from build123d import *

# Parameters (mm, degrees)
F0_W     = 45
F0_H     = 20
F1_DEPTH = 50
F3_SIZE  = 2
F4_SIZE  = 5
F2_R     = 5
F5_DEPTH = 45
F6_W     = 70
F6_H     = 70
F7_DEPTH = 50
F8_W     = 60
F8_H     = 60
F9_DEPTH = 40


with BuildPart() as f1:
    # F0 (on Top) → F1 (new body)
    with BuildSketch(Plane.XY):
        Rectangle(F0_W, F0_H)
    extrude(amount=F1_DEPTH)

    # F3
    f3_edges = [f1.edges().sort_by_distance(p)[0] for p in [
        (-22.5, -10, 25),
        (-22.5, 10, 25),
        (22.5, -10, 25),
        (22.5, 10, 25),
    ]]
    chamfer(f3_edges, length=F3_SIZE)

    # F4
    f4_edges = [f1.edges().sort_by_distance(p)[0] for p in [
        (0, 10, 0),
        (0, -10, 0),
    ]]
    chamfer(f4_edges, length=F4_SIZE)

    # F2 (on face) → F5 (cut, through all)
    with BuildSketch(Plane(origin=(-22.5, 0, 0), x_dir=(0, -1, 0), z_dir=(-1, 0, 0))):
        with Locations((0, 7)):
            Circle(F2_R)
    extrude(amount=-F5_DEPTH, mode=Mode.SUBTRACT)

    # F6 (on face) → F7 (join)
    with BuildSketch(Plane.XY.offset(50)):
        Rectangle(F6_W, F6_H)
    extrude(amount=F7_DEPTH)

    # F8 (on face) → F9 (cut)
    with BuildSketch(Plane.XY.offset(100)):
        Rectangle(F8_W, F8_H)
    extrude(amount=-F9_DEPTH, mode=Mode.SUBTRACT)


solid = f1.part
Could you check a few things on this model? Use its own coordinates, in mm. A direction names the side the tool comes from. Give positions to 0.01 mm unless a question says otherwise; leave off trailing zeros. Order: outer loops, then holes, each group sorted by start corner. A loop starts at its lowest first (then second) coordinate and runs counter-clockwise, first axis right, second up.
Item 1: If we section it at D-D, the plane y = -19: Write out the boundary of the cut face in (x, z).
Item 2: If we section it at B-B, the plane y = 0: Write out the boundary of the cut face in (x, z).
Item 3: If we section it at C-C, the plane x = -0.5: Write out the boundary of the cut face in (y, z), plus the area to 3 significant figures.
Item 4: I need wall thicknesses on line 1 (Z direction, x = -11, y = 0); line 2 (Y direction, x = -28, z = 79). Which ranges of each line are inside material? Lowest first, please.
Item 5: I'm going to push flat-ended pins straight in: pin 1 (1.5 mm diameter, centred on x = 20, y = 12, fed in from -Z); pin 2 (12 mm diameter, centred on x = 11, z = 30, fed in from +Y); pin 3 (10 mm diameter, centred on x = -21.5, y = -16, fed in from +Z); pin 4 (10 mm diameter, centred on x = 24.5, y = -1.5, fed in from -Z). Where does each tip first touch, or does it pass through?
Item 6: For faces 5 (the face through (22.5, 0, 25)), 6 (the face through (0, 30, 80)), 7 (the face through (0, -10, 27)), 8 (the face through (0, 10, 27)), which set-ups out of +Z, -Z, +X, -X, +Y, -Y let a thin tool reach every point of the face, with its end or its side?
Item 7: If we section it at A-A, the plane z = 7: Write out the boundary of the cut face in (x, y), plus the area to 3 significant figures.
Item 8: If we mould it in two halves opening along Y, with no side actions, what happens to faces 1 (the face through (0, 8, 3)), 2 (the face through (35, 0, 75)), 3 (the face through (0, -30, 80)), 4 (the face through (0, -8, 3))? For each: pulls with the +Y half, pulls with the -Y half, needs draft (parallel to the pull), parting line crosses it, or undercut.
Values:
1. outline: (-35, 50) - (35, 50) - (35, 100) - (30, 100) - (30, 60) - (-30, 60) - (-30, 100) - (-35, 100) - close
2. outline: (-35, 50) - (-22.5, 50) - (-22.5, 12) - (22.5, 12) - (22.5, 50) - (35, 50) - (35, 100) - (30, 100) - (30, 60) - (-30, 60) - (-30, 100) - (-35, 100) - close; (-22.5, 0) - (22.5, 0) - (22.5, 2) - (-22.5, 2) - close
3. outline: (-35, 50) - (-10, 50) - (-10, 5) - (-5, 0) - (5, 0) - (10, 5) - (10, 50) - (35, 50) - (35, 100) - (30, 100) - (30, 60) - (-30, 60) - (-30, 100) - (-35, 100) - close; hole circle Ø10 at (0, 7)
3. area: 2,000 mm2
4. line 1: z = 0 to 2, 12 to 60
4. line 2: y = -35 to -30, 30 to 35
5. pin 1: stops at z = 50
5. pin 2: stops at y = 10
5. pin 3: stops at z = 60
5. pin 4: stops at z = 0
6. face 5: -Z, +X, +Y, -Y
6. face 6: +Z
6. face 7: -Z, +X, -X, -Y
6. face 8: -Z, +X, -X, +Y
7. outline: (-22.5, -8) - (-20.5, -10) - (20.5, -10) - (22.5, -8) - (22.5, -5) - (-22.5, -5) - close; (-22.5, 5) - (22.5, 5) - (22.5, 8) - (20.5, 10) - (-20.5, 10) - (-22.5, 8) - close
7. area: 442 mm2
8. face 1: pulls with the +Y half
8. face 2: needs draft
8. face 3: undercut
8. face 4: pulls with the -Y half
